Source: three-view drawing plus pictorial views. Frame: mm from the lowest corner of the part. A direction names the side the tool comes from. Round coordinates to 2 decimals unless told otherwise and drop trailing zeros. Loops run counter-clockwise (first coordinate to the right, second up) from the corner with the lowest first, then second, coordinate; pieces in that order, holes last. Notation, with made-up numbers: M -27,-1 L 25,-1 A17 ccw 25,14 Z; hole C 76.25,32.5 d7. An arc over 180 degrees is marked long. Answer as a JSON object with one key per item and string values.
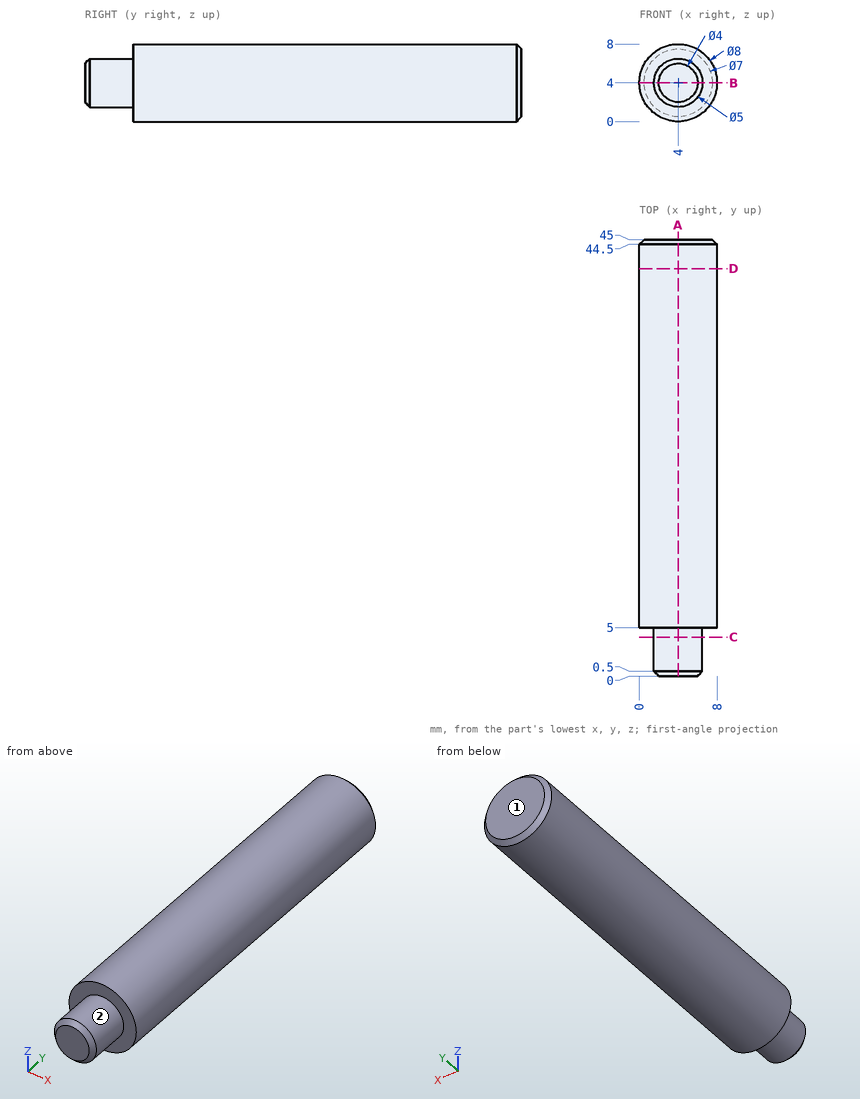
1) Set-up query: the marked faces 1 and 2. Return all of +Z, -Z, +X, -X, +Y, -Y with unobstructed straight access to the full face (end or side cutting, diameter ignored); none if empty.
Geometry results:
{"face 1": "+Z, -Z, +X, -X, +Y", "face 2": "-Y"}
2) Cut plane B-B on z = 4. Return the cut outline in (x, y).
Geometry results:
{"outline": "M 0,5 L 1.5,5 L 1.5,0.5 L 2,0 L 6,0 L 6.5,0.5 L 6.5,5 L 8,5 L 8,44.5 L 7.5,45 L 0.5,45 L 0,44.5 Z"}
3) Line query: probe 1 along Y at (x, z) = (1, 4.5); probe 2 along X at (y, z) = (30, 3.75); probe 3 along X at (y, z) = (43.5, 0.75). Output: solid intervals per line, ascending.
Geometry results:
{"probe 1": "5 to 45", "probe 2": "0.01 to 7.99", "probe 3": "1.67 to 6.33"}
4) Cut plane D-D on y = 42. Return the cut outline in (x, z).
Geometry results:
{"outline": "C 4,4 d8"}
5) Cut plane A-A on x = 4. Return the cut outline in (y, z), and give its area (4 significant figures).
Geometry results:
{"outline": "M 0,2 L 0.5,1.5 L 5,1.5 L 5,0 L 44.5,0 L 45,0.5 L 45,7.5 L 44.5,8 L 5,8 L 5,6.5 L 0.5,6.5 L 0,6 Z", "area": "344.5 mm2"}
6) First-contact query: pin 1 (3 mm diameter, centred on x = 6, z = 1, fed in from -Y); pin 2 (2 mm diameter, centred on x = 6.5, y = 13.5, fed in from +Z); pin 3 (1.5 mm diameter, centred on y = 6.5, z = 2.5, fed in from +X). Flat tips, straight axial feed; report the tip coordinate or a pass-through.
Geometry results:
{"pin 1": "y = 0.11", "pin 2": "z = 7.71", "pin 3": "x = 7.93"}
7) Cut plane C-C on y = 4. Return the cut outline in (x, z), and give its area (3 significant figures).
Geometry results:
{"outline": "C 4,4 d5", "area": "19.6 mm2"}
